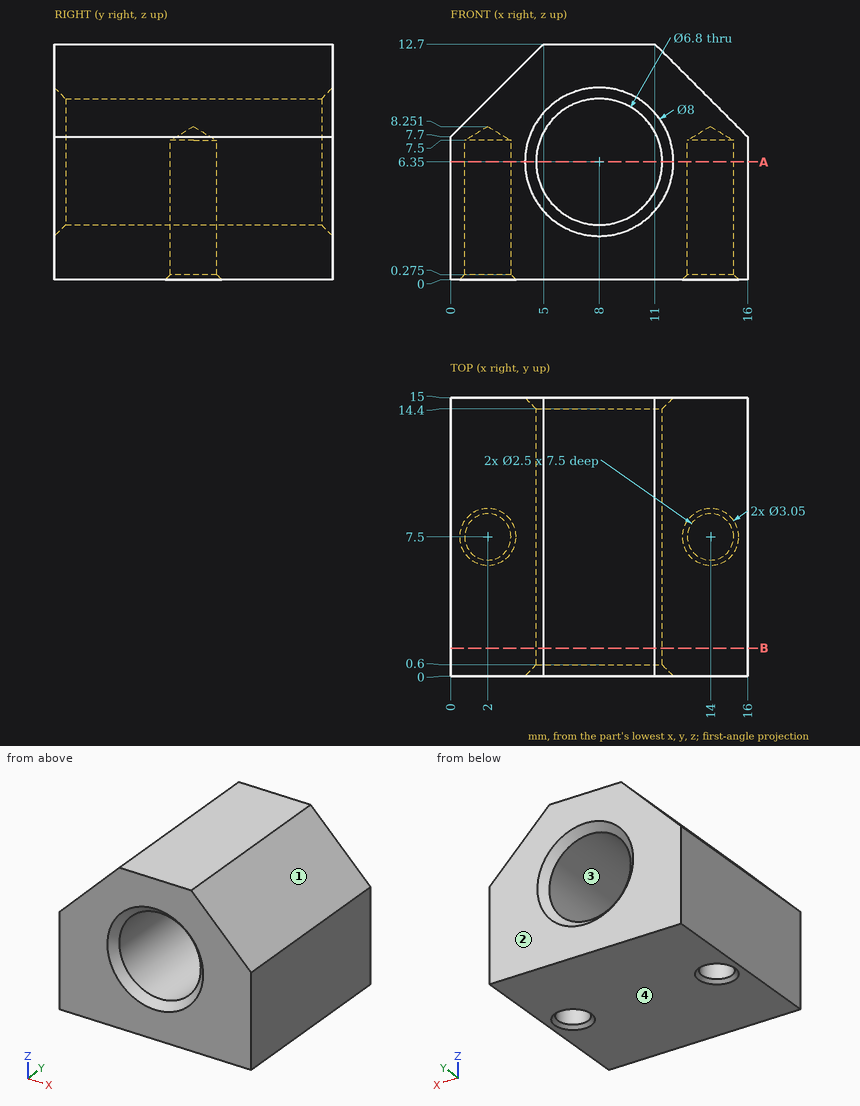
Check sheet for the drawn part. Datum: minimum x, y, z corner. Units: mm. Round coordinates to 2 decimals unless told otherwise and drop trailing zeros. Write each loop counter-clockwise with the first axis right and the second up, starting at its lowest first coordinate (ties: lowest second). Pieces come first, ordered by that corner, then holes. Notation, with made-up numbers: (31, 4.5) -> (39, 4.5) arc R29 cw to (39, 24.5) -> close; hole circle Ø7 at (-7.75, -31.75). An arc over 180 degrees is marked (long way). Write each question's results on one line, items separated by ' | '. Start each with the question number.
1. Depth check by flat-ended pin: P1, Ø2, axis at x = 14, y = 7.5, coming from the +Z side; P2, Ø4, axis at x = 2, y = 7.5, coming from the +Z side. Enter the tip coordinate at first touch or a pass-through.
2. Cross-section at A-A (z = 6.35). Enter the section's corners in (x, y).
3. Cross-section at B-B (y = 1.5). Enter the section's corners in (x, z).
4. Draft check along Z on the marked faces 1, 2, 3 and 4. Enter one of: +Z half, -Z half, draft (parallel to the pull), parting line (faces both ways), or undercut.
5. Material ranges on probe 1 along X at (y, z) = (5.75, 6.35); probe 2 along Y at (x, z) = (14, 3.5); probe 3 along Z at (x, y) = (8, 5.75), recorded low to high. Write a range as from..to.
Solutions:
1) P1: stops at z = 10.7 | P2: stops at z = 11.7
2) outline: (0, 0) -> (4, 0) -> (4.6, 0.6) -> (4.6, 14.4) -> (4, 15) -> (0, 15) -> close; (11.4, 0.6) -> (12, 0) -> (16, 0) -> (16, 15) -> (12, 15) -> (11.4, 14.4) -> close; hole circle Ø2.5 at (2, 7.5); hole circle Ø2.5 at (14, 7.5)
3) outline: (0, 0) -> (16, 0) -> (16, 7.7) -> (11, 12.7) -> (5, 12.7) -> (0, 7.7) -> close; hole circle Ø6.8 at (8, 6.35)
4) face 1: +Z half | face 2: draft | face 3: undercut | face 4: -Z half
5) probe 1: x = 0..4.6, 11.4..16 | probe 2: y = 0..6.25, 8.75..15 | probe 3: z = 0..2.95, 9.75..12.7
